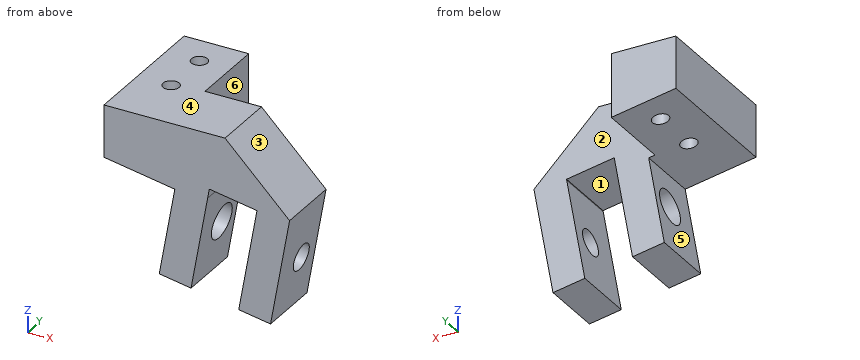
```python
from build123d import *

# Parameters (mm, degrees)
BOSS_EXTRU_1_DEPTH      = 10
BOSS_EXTRU_2_DEPTH      = 10
ENL_V_MAT_EXTRU_1_REACH = 37.367
ENL_V_MAT_EXTRU_2_REACH = 34.134
ESQUISSE4_R             = 2.75
ENL_V_MAT_EXTRU_3_REACH = 36.763
ESQUISSE5_R             = 2.1
CHANFREIN1_SIZE         = 10
ENL_V_MAT_EXTRU_4_REACH = 41.885
ENL_V_MAT_EXTRU_5_REACH = 47.008
ESQUISSE7_R             = 1.25


with BuildPart() as part:
    # Esquisse1 → Boss.-Extru.1 (new body)
    with BuildSketch(Plane.XY):
        Polygon((0, 0), (28.75, 0), (28.75, 10), (10, 10), (10, 22), (0, 22), align=None)
    extrude(amount=BOSS_EXTRU_1_DEPTH)

    # Esquisse2 → Boss.-Extru.2 (add)
    with BuildSketch(Plane(origin=(0, 10, 0), x_dir=(1, 0, 0), z_dir=(0, 1, 0))):
        Polygon((28.75, 0), (25.79798098, 16.741731801), (20.873942215, 15.873490913), (23.672866941, 0), align=None)
        Polygon((16.057167351, 0), (13.487884067, 14.57112958), (8.563845302, 13.702888692), (10.980034292, 0), align=None)
    extrude(amount=-BOSS_EXTRU_2_DEPTH)

    # Esquisse3 → Enlèv. mat.-Extru.1 (cut, up to next)
    with BuildSketch(Plane(origin=(0, 10, 0), x_dir=(1, 0, 0), z_dir=(0, 1, 0)), mode=Mode.PRIVATE) as enl_v_mat_extru_1_sk1:
        Polygon((16.057167351, 0), (16.317639618, -1.47721163), (23.703697766, -0.174850297), (23.672866941, 0), align=None)
    enl_v_mat_extru_1_tool1 = extrude(enl_v_mat_extru_1_sk1.sketch, amount=-ENL_V_MAT_EXTRU_1_REACH, mode=Mode.PRIVATE) & part.part
    add(enl_v_mat_extru_1_tool1.solids().sort_by_distance((18.952321, 10, 0.498572))[0], mode=Mode.SUBTRACT)

    # Esquisse4 → Enlèv. mat.-Extru.2 (cut, up to next)
    with BuildSketch(Plane(origin=(10.648945746, 0, -1.877696451), x_dir=(0.1736481776669311, 0, 0.9848077530122079), z_dir=(-0.9848077530122079, 0, 0.1736481776669311)), mode=Mode.PRIVATE) as enl_v_mat_extru_2_sk1:
        with Locations((-4.093337054, 6)):
            Circle(ESQUISSE4_R)
    enl_v_mat_extru_2_tool1 = extrude(enl_v_mat_extru_2_sk1.sketch, amount=-ENL_V_MAT_EXTRU_2_REACH, mode=Mode.PRIVATE) & part.part
    add(enl_v_mat_extru_2_tool1.solids().sort_by_distance((9.938145, 6, -5.908847))[0], mode=Mode.SUBTRACT)

    # Esquisse5 → Enlèv. mat.-Extru.3 (cut, up to next)
    with BuildSketch(Plane(origin=(22.959042659, 0, -4.048298672), x_dir=(0.1736481776669306, 0, 0.9848077530122081), z_dir=(-0.9848077530122081, 0, 0.1736481776669306)), mode=Mode.PRIVATE) as enl_v_mat_extru_3_sk1:
        with Locations((-4.093337054, 6)):
            Circle(ESQUISSE5_R)
    enl_v_mat_extru_3_tool1 = extrude(enl_v_mat_extru_3_sk1.sketch, amount=-ENL_V_MAT_EXTRU_3_REACH, mode=Mode.PRIVATE) & part.part
    add(enl_v_mat_extru_3_tool1.solids().sort_by_distance((22.248242, 6, -8.079449))[0], mode=Mode.SUBTRACT)

    # Chanfrein1
    chanfrein1_edges = [part.edges().sort_by_distance(p)[0] for p in [
        (28.75, 5, 10),
    ]]
    chamfer(chanfrein1_edges, length=CHANFREIN1_SIZE - 0.0001)  # a hair under: the kernel refuses the full size

    # Esquisse6 → Enlèv. mat.-Extru.4 (cut, up to next)
    with BuildSketch(Plane(origin=(0, 22, 0), x_dir=(1, 0, 0), z_dir=(0, 1, 0)), mode=Mode.PRIVATE) as enl_v_mat_extru_4_sk1:
        Polygon((0, 0), (10.980034292, 0), (0, -1.936076295), align=None)
    enl_v_mat_extru_4_tool1 = extrude(enl_v_mat_extru_4_sk1.sketch, amount=-ENL_V_MAT_EXTRU_4_REACH, mode=Mode.PRIVATE) & part.part
    add(enl_v_mat_extru_4_tool1.solids().sort_by_distance((3.660011, 22, 0.645359))[0], mode=Mode.SUBTRACT)

    # Enlèv. mat.-Extru.5: up to this plane
    enl_v_mat_extru_5_end = Plane(origin=(10.980034292, -0.001, 0), z_dir=(0.17364817766693136, 0, 0.9848077530122079))
    # Esquisse7 → Enlèv. mat.-Extru.5 (cut, up to the surface)
    with BuildSketch(Plane.XY.offset(10), mode=Mode.PRIVATE) as enl_v_mat_extru_5_sk1:
        with Locations((5.19, 17)):
            Circle(ESQUISSE7_R)
    enl_v_mat_extru_5_tool1 = split(extrude(enl_v_mat_extru_5_sk1.sketch, amount=-ENL_V_MAT_EXTRU_5_REACH, mode=Mode.PRIVATE), bisect_by=enl_v_mat_extru_5_end, keep=Keep.BOTH, mode=Mode.PRIVATE)
    add(enl_v_mat_extru_5_tool1.solids().sort_by_distance((5.19, 17, 10))[0], mode=Mode.SUBTRACT)
    # Esquisse7 → Enlèv. mat.-Extru.5 (cut, up to the surface)
    with BuildSketch(Plane.XY.offset(10), mode=Mode.PRIVATE) as enl_v_mat_extru_5_sk2:
        with Locations((5.19, 9.22)):
            Circle(ESQUISSE7_R)
    enl_v_mat_extru_5_tool2 = split(extrude(enl_v_mat_extru_5_sk2.sketch, amount=-ENL_V_MAT_EXTRU_5_REACH, mode=Mode.PRIVATE), bisect_by=enl_v_mat_extru_5_end, keep=Keep.BOTH, mode=Mode.PRIVATE)
    add(enl_v_mat_extru_5_tool2.solids().sort_by_distance((5.19, 9.22, 10))[0], mode=Mode.SUBTRACT)


solid = part.part
```
Geometry check sheet. Reference: the model listing, model coordinates, mm. Face numbers are marked on the shaded views. A direction names the side the tool comes from. Give positions to 0.01 mm unless a question says otherwise; leave off trailing zeros. Write each loop counter-clockwise with the first axis right and the second up, starting at its lowest first coordinate (ties: lowest second). Pieces come first, ordered by that corner, then holes. Notation, with made-up numbers: (-37.75, -31) -> (-13.75, -31) arc R14 ccw to (-13.75, -8) -> close; hole circle Ø1 at (67, -3). An arc over 180 degrees is marked (long way). One line per question, with ' | ' between items.
Item 1: Depth check by flat-ended pin: pin 1 (4 mm diameter, centred on x = 11, y = 10.5, fed in from -Z); pin 2 (1.5 mm diameter, centred on y = 10, z = 5, fed in from +X); pin 3 (1 mm diameter, centred on x = 5.5, y = 10.5, fed in from -Z). Enter the tip coordinate at first touch or a pass-through.
Determined:
pin 1: z = -14.47 | pin 2: x = 24.5 | pin 3: z = 0.88
Item 2: Access from +Z, -Z, +X, -X, +Y, -Y to the whole of each face (thin tool, end or side, straight path). Record for the marked faces 4, 5 and 6.
Determined:
face 4: +Z, +X, -X, +Y, -Y | face 5: -X, +Y, -Y | face 6: +Z, -Z, +X, +Y
Item 3: Sectioned sample at B-B, the plane z = 7. Record the boundary of the cut face in (x, y).
Determined:
outline: (0, 0) -> (21.75, 0) -> (21.75, 10) -> (10, 10) -> (10, 22) -> (0, 22) -> close; hole circle Ø2.5 at (5.19, 9.22); hole circle Ø2.5 at (5.19, 17)
Item 4: Scan lines: line 1 along Y through (x, z) = (5.19, 7); line 2 along X through (y, z) = (17, 3.5); line 3 along Y through (x, z) = (6, 6.25). Record each from-to range of solid material in increasing order.
Determined:
line 1: 0 to 7.97, 10.47 to 15.75, 18.25 to 22 | line 2: 0 to 3.94, 6.44 to 10 | line 3: 0 to 8.27, 10.17 to 16.05, 17.95 to 22
Item 5: Sectioned sample at C-C, the plane x = 21.5. Record the boundary of the cut face in (y, z), plus the area to 3 significant figures.
Determined:
outline: (0, -15.98) -> (10, -15.98) -> (10, -12.32) -> (0, -12.32) -> close; (0, 0.56) -> (10, 0.56) -> (10, 7.25) -> (0, 7.25) -> close | area: 103 mm^2
Item 6: Sectioned sample at A-A, the plane y = 7.5. State how many separate pieces and enclosed holes the cut face has, plus the area to 3 significant figures.
Determined:
separate pieces: 3 | enclosed holes: 0 | area: 337 mm^2
Item 7: Draft check along Z on the marked faces 1, 2 and 3. Enter one of: released by +Z, released by -Z, zero draft, split by the parting line, or undercut.
Determined:
face 1: undercut | face 2: zero draft | face 3: released by +Z
Item 8: Sectioned sample at D-D, the plane z = -1. Record the boundary of the cut face in (x, y).
Determined:
outline: (10.8, 0) -> (15.88, 0) -> (15.88, 10) -> (10.8, 10) -> close; (23.5, 0) -> (28.57, 0) -> (28.57, 10) -> (23.5, 10) -> close
